Autodesk Inventor part; units mm, degrees
ref_plane "YZ Plane" through (0, 0, 0) normal (1, 0, 0) x (0, 1, 0)
ref_plane "XZ Plane" through (0, 0, 0) normal (0, 1, 0) x (-1, 0, 0)
ref_plane "XY Plane" through (0, 0, 0) normal (0, 0, 1) x (1, 0, 0)
sketch "Sketch1" plane through (0, 0, 0) normal (0, 1, 0) x (-1, 0, 0)
  circle A0 centre (0, 0) radius 10 construction
  line L0 (10, 0) -> (5, -8.6603)
  line L1 (5, -8.6603) -> (-5, -8.6603)
  line L2 (-5, -8.6603) -> (-10, 0)
  line L3 (-10, 0) -> (-5, 8.6603)
  line L4 (-5, 8.6603) -> (5, 8.6603)
  line L5 (5, 8.6603) -> (10, 0)
  circle A1 centre (0, 0) radius 5
  dimension "d0" = 20
  dimension "d3" = 10
extrude "Extrusion1" add sketch "Sketch1" along normal blind 10 contours L0 L1 L2 L3 L4 L5 | A1
extrude "Extrusion2" cut sketch "Sketch1" along normal blind 10 contours A1
thread "Thread1"
properties part number "NutA" material "Titanium"
CAD build for the part. Positions are in the model's coordinates, mm. Coordinates: 2 decimals unless noted, no trailing zeros. Loops run counter-clockwise (first coordinate to the right, second up) from the corner with the lowest first, then second, coordinate; pieces in that order, holes last. Notation, with made-up numbers: (-2.5, 88.25) - (37.5, 88.25) arc R29 cw to (37.5, 111.25) - close; hole circle Ø7 at (-38, 23). An arc over 180 degrees is marked (long way). Return JSON: item names as keys, results as strings.
1. Drop flat-ended pins along their axis: pin 1 (1 mm diameter, centred on y = 2.5, z = -1.5, fed in from +X); pin 2 (1 mm diameter, centred on y = 6.5, z = 6, fed in from -X); pin 3 (1 mm diameter, centred on y = 5.5, z = 1, fed in from -X). Give the stop position or say it passes through.
Result:
{"pin 1": "stops at x = 9.42", "pin 2": "stops at x = -6.82", "pin 3": "stops at x = -9.71"}
2. Band-saw the part on B-B (y = 4.75). Give the cut face in (x, z), and give its area (3 significant figures).
Result:
{"outline": "(-10, 0) - (-5, -8.66) - (5, -8.66) - (10, 0) - (5, 8.66) - (-5, 8.66) - close; hole circle Ø10 at (0, 0)", "area": "181 mm2"}
3. Band-saw the part on C-C (z = 2). Give the cut face in (x, y).
Result:
{"outline": "(-8.85, 0) - (-4.58, 0) - (-4.58, 10) - (-8.85, 10) - close; (4.58, 0) - (8.85, 0) - (8.85, 10) - (4.58, 10) - close"}
4. Band-saw the part on D-D (z = 5.75). Give the cut face in (x, y).
Result:
{"outline": "(-6.68, 0) - (6.68, 0) - (6.68, 10) - (-6.68, 10) - close"}
5. Band-saw the part on A-A (x = 3). Give the cut face in (y, z), and give its area (3 significant figures).
Result:
{"outline": "(0, -8.66) - (10, -8.66) - (10, -4) - (0, -4) - close; (0, 4) - (10, 4) - (10, 8.66) - (0, 8.66) - close", "area": "93.2 mm2"}
6. Mould opens along Z. For faces 1 (the flat face through (-4, 10, 4)), 2 (the flat face through (-7.465, 4.93, 4.391)), 3 (the cylindrical face through (1.08, 4.93, 4.88)) say: released by +Z, released by -Z, zero draft, split by the parting line, or undercut.
Result:
{"face 1": "zero draft", "face 2": "released by +Z", "face 3": "undercut"}
7. Probe L1, parallel to Z at x = 0, y = 4.75; L2, parallel to X at y = 3.5, z = -2.75; L3, parallel to X at y = 6, z = 0.5. List the from-to ranges inside material, lowest first. Write a range as from..to.
Result:
{"L1": "z = -8.66..-5, 5..8.66", "L2": "x = -8.41..-4.18, 4.18..8.41", "L3": "x = -9.71..-4.97, 4.97..9.71"}
